Geometry check sheet. Reference: the model listing, model coordinates, mm. A direction names the side the tool comes from. Round coordinates to 2 decimals unless told otherwise and drop trailing zeros. Write each loop counter-clockwise with the first axis right and the second up, starting at its lowest first coordinate (ties: lowest second). Pieces come first, ordered by that corner, then holes. Notation, with made-up numbers: (-17.75, 41.25) - (26.25, 41.25) arc R18 cw to (26.25, 75.25) - close; hole circle Ø10 at (30, 60.5). An arc over 180 degrees is marked (long way). Return JSON: item names as keys, results as strings.
```python
from build123d import *

# Parameters (mm, degrees)
SKETCH040_W    = 252
SKETCH040_H    = 268
PAD011_DEPTH   = 55
FILLET013_R    = 6
THICKNESS001_T = 3


with BuildPart() as part:
    # Sketch040 → Pad011 (new body)
    with BuildSketch(Plane.XY):
        with Locations((0, -134)):
            Rectangle(SKETCH040_W, SKETCH040_H)
    extrude(amount=PAD011_DEPTH)

    # Fillet013
    fillet013_edges = [part.edges().sort_by_distance(p)[0] for p in [
        (126, -268, 27.5),
        (-126, -268, 27.5),
    ]]
    fillet(fillet013_edges, radius=FILLET013_R)

    # Thickness001
    thickness001_openings = [part.faces().sort_by_distance(p)[0] for p in [
        (0, -133.969642, 55),
        (0, -133.969642, 0),
        (0, 0, 27.5),
    ]]
    offset(amount=THICKNESS001_T, openings=thickness001_openings)


solid = part.part
```
(1) Material ranges on line 1 along X through (y, z) = (-119.5, 32.5); line 2 along Y through (x, z) = (-57.5, 3.5), recorded low to high. Write a range as [from, to].
Response values:
{"line 1": "x = [-129, -126], [126, 129]", "line 2": "y = [-271, -268]"}
(2) Section check B-B, the plane z = 21. Enter the section's corners in (x, y).
Response values:
{"outline": "(-129, -262) arc R9 ccw to (-120, -271) - (120, -271) arc R9 ccw to (129, -262) - (129, 0) - (126, 0) - (126, -262) arc R6 cw to (120, -268) - (-120, -268) arc R6 cw to (-126, -262) - (-126, 0) - (-129, 0) - close"}
(3) Section check A-A, the plane y = -71. Enter the section's corners in (x, z), plus the area to 3 significant figures.
Response values:
{"outline": "(-129, 0) - (-126, 0) - (-126, 55) - (-129, 55) - close; (126, 0) - (129, 0) - (129, 55) - (126, 55) - close", "area": "330 mm^2"}
(4) Release check for a two-part mould opening along X. For faces 1 (the face through (-129, -133, 27)), 2 (the face through (-2, -271, 27)), 3 (the face through (-124.289, -266.196, 27.885)), 4 (the face through (126.294, -268.434, 27.885)) record: pulls with the +X half, pulls with the -X half, needs draft (parallel to the pull), parting line crosses it, or undercut.
Response values:
{"face 1": "pulls with the -X half", "face 2": "needs draft", "face 3": "undercut", "face 4": "pulls with the +X half"}
(5) Section check C-C, the plane x = 111. Enter the section's corners in (y, z).
Response values:
{"outline": "(-271, 0) - (-268, 0) - (-268, 55) - (-271, 55) - close"}
(6) Gauge pin test, flat end, axial feed: pin 1 (16.5 mm diameter, centred on x = -2.5, z = 20.5, fed in from +Y). Record the tip position at first contact, or that the pin passes through.
Response values:
{"pin 1": "stops at y = -268"}
(7) Access from +Z, -Z, +X, -X, +Y, -Y to the whole of each face (thin tool, end or side, straight path). Record for faces 5 (the face through (-126.434, -268.294, 27.885)), 6 (the face through (124.196, -266.289, 27.885)).
Response values:
{"face 5": "+Z, -Z, -X, -Y", "face 6": "+Z, -Z, +Y"}
